Geometry check sheet. Reference: the model listing, model coordinates, mm. Face numbers are marked on the shaded views. A direction names the side the tool comes from. Coordinates: 2 decimals unless noted, no trailing zeros. Order: outer loops, then holes, each group sorted by start corner. A loop starts at its lowest first (then second) coordinate and runs counter-clockwise, first axis right, second up. Notation, with made-up numbers: (12.25, 22.5) - (67.25, 22.5) arc R25 cw to (67.25, 35.5) - close; hole circle Ø3 at (88.25, 26.5). An arc over 180 degrees is marked (long way). Put each result on its own line as item: value.
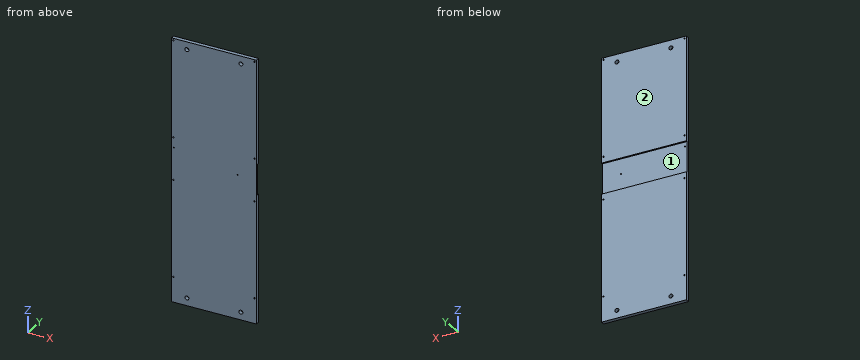
from build123d import *

# Parameters (mm, degrees)
SKETCH1_W           = 139.7
SKETCH1_H           = 431.8
BOSS_EXTRUDE1_DEPTH = 6.35
SKETCH3_R           = 1.1303
CUT_EXTRUDE6_DEPTH  = 6.35
SKETCH4_W           = 139.7
SKETCH4_H           = 50.8
CUT_EXTRUDE7_DEPTH  = 2.54
SKETCH5_R           = 0.889
CUT_EXTRUDE8_DEPTH  = 454.852229365
SKETCH6_R           = 3.2639
CUT_EXTRUDE9_DEPTH  = 454.880658874


with BuildPart() as part:
    # Sketch1 → Boss-Extrude1 (new body)
    with BuildSketch(Plane(origin=(0, 0, 0), x_dir=(1, 0, 0), z_dir=(0, 1, 0))):
        with Locations((69.85, 215.9)):
            Rectangle(SKETCH1_W, SKETCH1_H)
    extrude(amount=BOSS_EXTRUDE1_DEPTH)

    # Sketch3 → Cut-Extrude6 (cut)
    with BuildSketch(Plane(origin=(0, 6.35, 0), x_dir=(1, 0, 0), z_dir=(0, 1, 0))):
        with Locations(Location((3.175, 3.175, 0), (0, 0, 270))):
            Circle(SKETCH3_R)
        with Locations(Location((136.525, 3.175, 0), (0, 0, 270))):
            Circle(SKETCH3_R)
        with Locations(Location((136.525, 161.925, 0), (0, 0, 90))):
            Circle(SKETCH3_R)
        with Locations(Location((136.525, 231.775, 0), (0, 0, 270))):
            Circle(SKETCH3_R)
        with Locations(Location((3.175, 161.925, 0), (0, 0, 270))):
            Circle(SKETCH3_R)
        with Locations(Location((3.175, 231.775, 0), (0, 0, 90))):
            Circle(SKETCH3_R)
        with Locations(Location((3.175, 390.525, 0), (0, 0, 90))):
            Circle(SKETCH3_R)
        with Locations(Location((136.525, 390.525, 0), (0, 0, 270))):
            Circle(SKETCH3_R)
    extrude(amount=-CUT_EXTRUDE6_DEPTH, mode=Mode.SUBTRACT)

    # Sketch4 → Cut-Extrude7 (cut)
    with BuildSketch(Plane(origin=(0, 6.35, 0), x_dir=(1, 0, 0), z_dir=(0, 1, 0))):
        with Locations((69.85, 196.85)):
            Rectangle(SKETCH4_W, SKETCH4_H)
    extrude(amount=-CUT_EXTRUDE7_DEPTH, mode=Mode.SUBTRACT)

    # Sketch5 → Cut-Extrude8 (cut, through all)
    with BuildSketch(Plane(origin=(0, 3.81, 0), x_dir=(1, 0, 0), z_dir=(0, 1, 0))):
        with Locations(Location((3.81, 178.816, 0), (0, 0, 270))):
            Circle(SKETCH5_R)
        with Locations(Location((108.966, 195.834, 0), (0, 0, 270))):
            Circle(SKETCH5_R)
    extrude(amount=-CUT_EXTRUDE8_DEPTH, mode=Mode.SUBTRACT)

    # Sketch6 → Cut-Extrude9 (cut, through all)
    with BuildSketch(Plane(origin=(0, 6.35, 0), x_dir=(1, 0, 0), z_dir=(0, 1, 0))):
        with Locations(Location((25.4, 419.1, 0), (0, 0, 270))):
            Circle(SKETCH6_R)
        with Locations(Location((114.3, 419.1, 0), (0, 0, 90))):
            Circle(SKETCH6_R)
        with Locations(Location((114.3, 12.7, 0), (0, 0, 270))):
            Circle(SKETCH6_R)
        with Locations(Location((25.4, 12.7, 0), (0, 0, 90))):
            Circle(SKETCH6_R)
    extrude(amount=-CUT_EXTRUDE9_DEPTH, mode=Mode.SUBTRACT)


solid = part.part
Q1. Section check A-A on y = 5. State how many separate pieces and enclosed holes the cut face has, then the cut area to 3 significant figures.
Answer block:
separate pieces: 2
enclosed holes: 12
area: 53,100 mm^2
Q2. Access from +Z, -Z, +X, -X, +Y, -Y to the whole of each face (thin tool, end or side, straight path). Record for the marked faces 1 and 2.
Answer block:
face 1: +X, -X, +Y
face 2: +Z, -Z, +X, -X, +Y
Q3. Depth check by flat-ended pin: pin 1 Ø1.4 at (x, z) = (108.966, -195.834) entering from -Y; pin 2 Ø10.5 at (x, z) = (25.4, -419.1) entering from +Y; pin 3 Ø15 at (x, z) = (82.5, -197) entering from +Y. Enter the tip coordinate at first touch or a pass-through.
Answer block:
pin 1: passes through
pin 2: stops at y = 6.35
pin 3: stops at y = 3.81
Q4. Thickness scan on L1, parallel to X at y = 3.25, z = -12.7; L2, parallel to Z at x = 74.5, y = 5.25; L3, parallel to Y at x = 12.5, z = -209.5. Record the ranges inside material, lowest first. Write a range as [from, to].
Answer block:
L1: x = [0, 22.14], [28.66, 111.04], [117.56, 139.7]
L2: z = [-431.8, -222.25], [-171.45, 0]
L3: y = [0, 3.81]
Q5. Section check B-B on x = 65. Record the boundary of the cut face in (y, z), then the cut area to 3 significant figures.
Answer block:
outline: (0, -431.8) - (6.35, -431.8) - (6.35, -222.25) - (3.81, -222.25) - (3.81, -171.45) - (6.35, -171.45) - (6.35, 0) - (0, 0) - close
area: 2,610 mm^2
